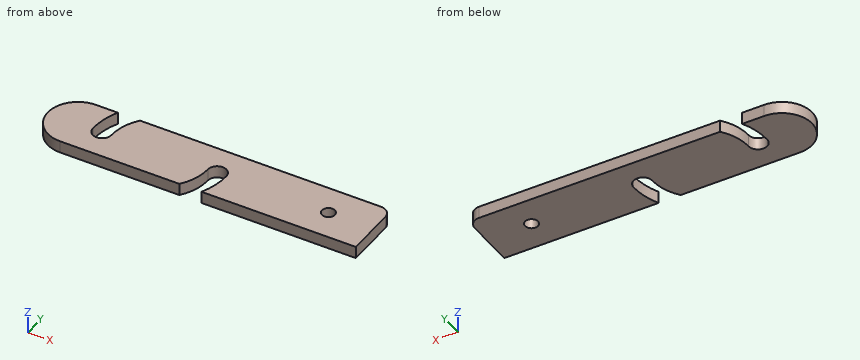
```python
from build123d import *

# Parameters (mm, degrees)
SKETCH1_R           = 2.15
BOSS_EXTRUDE1_DEPTH = 4


with BuildPart() as part:
    # Sketch1 → Boss-Extrude1 (new body)
    with BuildSketch(Plane.XY):
        with BuildLine():
            Line((20.7866022, -13), (-18.694986916, -13))
            ThreePointArc((-18.694986916, -13), (-28.694986916, -3), (-18.694986916, 7))
            Line((-18.694986916, 7), (-11.409460793, 7))
            ThreePointArc((-11.409460793, 7), (-13.190353922, 2.140299964), (-13.794986916, -3))
            ThreePointArc((-13.794986916, -3), (-10.694986916, -6.1), (-7.594986916, -3))
            ThreePointArc((-7.594986916, -3), (-6.688371741, 2.301283436), (-4.071576031, 7))
            Line((-4.071576031, 7), (75.805013084, 7))
            ThreePointArc((75.805013084, 7), (78.279886819, 5.974873734), (79.305013084, 3.5))
            Line((79.305013084, 3.5), (79.305013084, -13))
            Line((79.305013084, -13), (28.124486961, -13))
            ThreePointArc((28.124486961, -13), (29.905380091, -8.140299964), (30.510013084, -3))
            ThreePointArc((30.510013084, -3), (27.410013084, 0.1), (24.310013084, -3))
            ThreePointArc((24.310013084, -3), (23.40339791, -8.301283436), (20.7866022, -13))
        make_face()
        with Locations((64.305013084, -3)):
            Circle(SKETCH1_R, mode=Mode.SUBTRACT)
    extrude(amount=BOSS_EXTRUDE1_DEPTH)


solid = part.part
```
The model under review builds one solid part; all positions refer to its coordinate system, in mm. Give positions to 0.01 mm unless a question says otherwise; leave off trailing zeros. Write each loop counter-clockwise with the first axis right and the second up, starting at its lowest first coordinate (ties: lowest second). Pieces come first, ordered by that corner, then holes. Notation, with made-up numbers: (-8, 47.5) -> (46, 47.5) arc R36 ccw to (46, 82.5) -> close; hole circle Ø8 at (29.5, -20.75). An arc over 180 degrees is marked (long way). Answer in a Markdown table with one row per item.
1) Clearance check with flat-ended pins moving along their axes: P1, Ø4, axis at x = 64.31, y = -3, coming from the -Z side; P2, Ø1, axis at y = -6.5, z = 3, coming from the -X side. State where each tip first meets the part, or that it passes through.
Worked answers:
| item | result |
|---|---|
| P1 | through |
| P2 | x = -28.23 |
2) For L1, parallel to X at y = -0.5, z = 0.45; L2, parallel to X at y = -8.25, z = 3.2; L3, parallel to X at y = 1.5, z = 0.4, list the stretches that pass through material, from the lowest coordinate up. Write a range as [from, to].
Worked answers:
| item | result |
|---|---|
| L1 | [-28.38, -13.65], [-7.4, 25.58], [29.24, 79.31] |
| L2 | [-27.21, 23.42], [29.88, 79.31] |
| L3 | [-27.63, -13.33], [-6.95, 79.31] |
3) Add section D-D on x = -5.5. State the section outline as (y, z) points.
Worked answers:
| item | result |
|---|---|
| outline | (-13, 0) -> (4.9, 0) -> (4.9, 4) -> (-13, 4) -> close |
4) Add section B-B on y = -9. State the section outline as (x, z) points.
Worked answers:
| item | result |
|---|---|
| outline | (-26.69, 0) -> (23.14, 0) -> (23.14, 4) -> (-26.69, 4) -> close; (29.68, 0) -> (79.31, 0) -> (79.31, 4) -> (29.68, 4) -> close |
5) Add section C-C on y = 1. State the section outline as (x, z) points, plus the area to 3 significant figures.
Worked answers:
| item | result |
|---|---|
| outline | (-27.86, 0) -> (-13.43, 0) -> (-13.43, 4) -> (-27.86, 4) -> close; (-7.09, 0) -> (79.31, 0) -> (79.31, 4) -> (-7.09, 4) -> close |
| area | 403 mm² |
